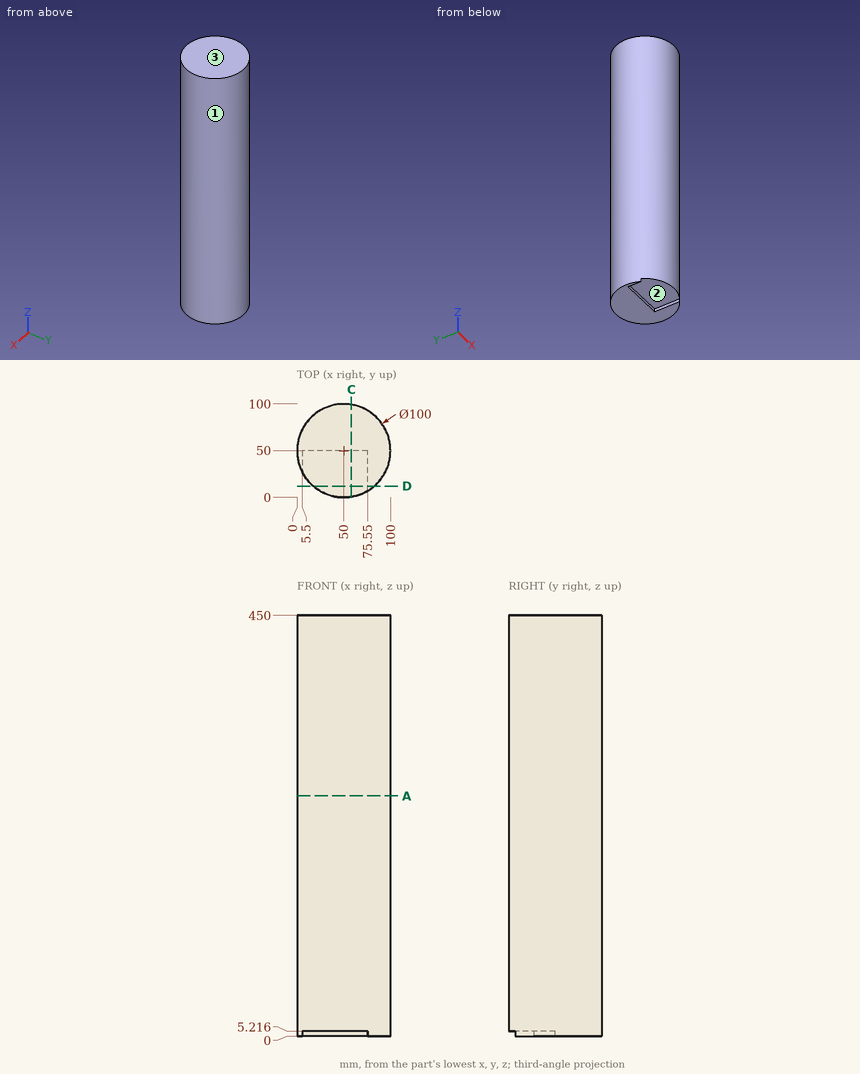
Job drawing, mm, ordinate dimensions from the low corner. One solid piece. Give positions to 0.01 mm unless a question says otherwise; leave off trailing zeros. Order: outer loops, then holes, each group sorted by start corner. A loop starts at its lowest first (then second) coordinate and runs counter-clockwise, first axis right, second up. Notation, with made-up numbers: (-18, 3.5) - (1, 3.5) arc R33 ccw to (1, 36.5) - close; hole circle Ø6 at (73, -3). An arc over 180 degrees is marked (long way). Answer in a Markdown table with one row per item.
1. Saw through at A-A, the plane z = 257. Give the cut face in (x, y), plus the area to 3 significant figures.
Data:
| item | result |
|---|---|
| outline | circle Ø100 at (50, 50) |
| area | 7,850 mm² |
2. Flat gauge pins, fed straight in: pin 1 (15 mm diameter, centred on x = 25.5, y = 15, fed in from -Z); pin 2 (6 mm diameter, centred on x = 85, z = 363, fed in from -Y); pin 3 (5.5 mm diameter, centred on y = 41, z = 3.5, fed in from +X); pin 4 (5 mm diameter, centred on x = 71.5, y = 87, fed in from -Z). Where does each tip first touch, or does it go through?
Data:
| item | result |
|---|---|
| pin 1 | stops at z = 5.22 |
| pin 2 | stops at y = 11.58 |
| pin 3 | stops at x = 99.61 |
| pin 4 | stops at z = 0 |
3. Saw through at C-C, the plane x = 58. Give the cut face in (y, z) (1 decimal).
Data:
| item | result |
|---|---|
| outline | (0.6, 5.2) - (50, 5.2) - (50, 0) - (99.4, 0) - (99.4, 450) - (0.6, 450) - close |
4. Probe probe 1 along Z at (x, y) = (58.5, 24); probe 2 along X at (y, z) = (76.5, 91.5); probe 3 along X at (y, z) = (46, 106.5). List the from-to ranges inside material, lowest first. Write a range as [from, to].
Data:
| item | result |
|---|---|
| probe 1 | z = [5.22, 450] |
| probe 2 | x = [7.6, 92.4] |
| probe 3 | x = [0.16, 99.84] |
5. Saw through at D-D, the plane y = 12. Give the cut face in (x, z), plus the area to 3 significant figures.
Data:
| item | result |
|---|---|
| outline | (17.5, 5.22) - (75.55, 5.22) - (75.55, 0) - (82.5, 0) - (82.5, 450) - (17.5, 450) - close |
| area | 28,900 mm² |
6. Pull direction X, two halves, no side cores. Call the marked faces 1, 2 and 3: pulls with the +X half, pulls with the -X half, needs draft (parallel to the pull), parting line crosses it, or undercut.
Data:
| item | result |
|---|---|
| face 1 | parting line crosses it |
| face 2 | undercut |
| face 3 | needs draft |
